Verification items for this drawing (mm, ordinates from the low corner). Give positions to 0.01 mm unless a question says otherwise; leave off trailing zeros. Order: outer loops, then holes, each group sorted by start corner. A loop starts at its lowest first (then second) coordinate and runs counter-clockwise, first axis right, second up.
(1) Sectioned sample at B-B on z = 12.5. Count the separate pieces of the cut face and the enclosed holes in it.
(2) Scan lines: L1, parallel to Y at x = 5.4, z = 8.75; L2, parallel to X at y = 5.25, z = 1.25; L3, parallel to Y at x = 7.5, z = 6 (1 decimal). Record each from-to range of solid material in increasing order.
(3) Gauge pin test, flat ends, axial feed: pin 1 (1 mm diameter, centred on x = 4, y = 2.5, fed in from -Z); pin 2 (3 mm diameter, centred on x = 8.5, z = 2, fed in from -Y). Record the tip position at first contact, or that the pin passes through.
(4) Mould release check, pull along Y, two halves, no side actions. Record for the marked faces 1, 2 and 3: pulls with the +Y half, pulls with the -Y half, needs draft (parallel to the pull), parting line crosses it, or undercut.
(5) Sectioned sample at A-A on y = 5.4. Record the cut outline in (x, z).
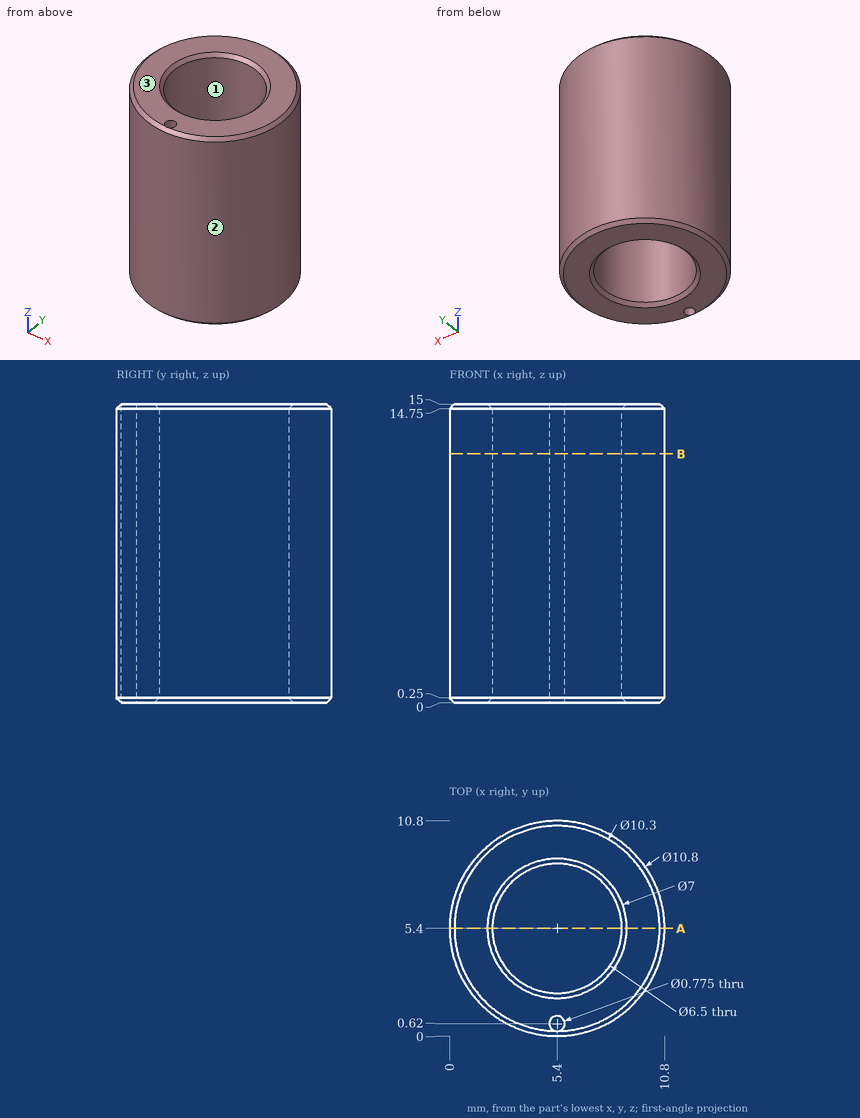
Ans:
1. separate pieces: 1
1. enclosed holes: 2
2. L1: y = 0 to 0.23, 1.01 to 2.15, 8.65 to 10.8
2. L2: x = 0 to 2.15, 8.65 to 10.8
2. L3: y = 0.4 to 2.9, 7.9 to 10.4
3. pin 1: stops at z = 0
3. pin 2: stops at y = 0.24
4. face 1: undercut
4. face 2: parting line crosses it
4. face 3: needs draft
5. outline: (0, 0.25) - (0.25, 0) - (1.9, 0) - (2.15, 0.25) - (2.15, 14.75) - (1.9, 15) - (0.25, 15) - (0, 14.75) - close; (8.65, 0.25) - (8.9, 0) - (10.55, 0) - (10.8, 0.25) - (10.8, 14.75) - (10.55, 15) - (8.9, 15) - (8.65, 14.75) - close
